Could you check a few things on this drawing? It's one solid part, dimensions in mm from its lowest x, y, z. A direction names the side the tool comes from. Round coordinates to 2 decimals unless told otherwise and drop trailing zeros. Write each loop counter-clockwise with the first axis right and the second up, starting at its lowest first coordinate (ties: lowest second). Pieces come first, ordered by that corner, then holes. Notation, with made-up numbers: (45, -35.75) -> (86, -35.75) arc R9 cw to (86, -31.75) -> close; hole circle Ø7 at (20, 71.25). An arc over 180 degrees is marked (long way). Put each result on its own line as item: value. Start each with the question number.
1) Which directions (+Z, -Z, +X, -X, +Y, -Y) give clear straight access to the entire face, cutting with the end or side of a thin tool? Please do the marked faces 1 and 2.
2) I want a section at C-C, the plane z = 5.25. List the corners of the cut face in (x, y) for me.
3) I want a section at A-A, the plane y = 5. List the corners of the cut face in (x, z) for me, then the cut area to 3 significant figures.
4) If I drill on line 1 along Z through (x, y) = (7, 8.5); line 2 along X through (y, z) = (2.5, 5.75); line 3 along Y through (x, z) = (3.5, 5), over which ranges is the centre line in solid material (lowest first)? Write a range as [from, to].
5) Will these pins go through, and if not, where does the flat tip stop? P1, Ø4, axis at x = 2, y = 8, coming from the -Z side; P2, Ø1, axis at x = 7, z = 1.5, coming from the +Y side.
6) I want a section at D-D, the plane y = 9. List the corners of the cut face in (x, z) for me.
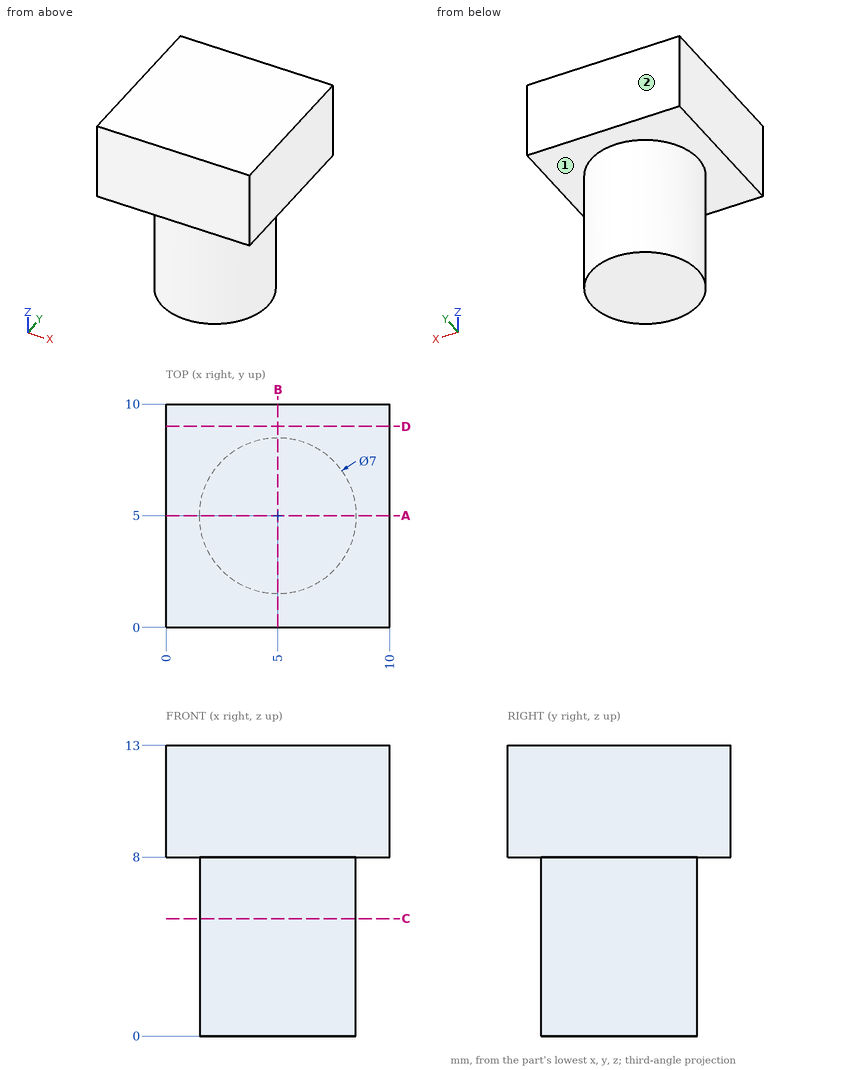
Findings:
1. face 1: -Z
1. face 2: +Z, -Z, +X, -X, +Y
2. outline: circle Ø7 at (5, 5)
3. outline: (0, 8) -> (1.5, 8) -> (1.5, 0) -> (8.5, 0) -> (8.5, 8) -> (10, 8) -> (10, 13) -> (0, 13) -> close
3. area: 106 mm2
4. line 1: z = [8, 13]
4. line 2: x = [2.55, 7.45]
4. line 3: y = [1.84, 8.16]
5. P1: stops at z = 0
5. P2: stops at y = 8.16
6. outline: (0, 8) -> (10, 8) -> (10, 13) -> (0, 13) -> close
